Can you work these out from the model? Positions are in its coordinate system, mm. A direction names the side the tool comes from. Coordinates: 2 decimals unless noted, no trailing zeros. Use one line per item in the form item = value.
```python
from build123d import *

# Parameters (mm, degrees)
F0_R     = 1.6
F0_R_2   = 1.25
F0_R_3   = 2
F0_R_4   = 3
F1_DEPTH = 3.175


# Not quite as in the source:
# - a feature names something its author has since deleted; it is built from what else it names


with BuildPart() as f1:
    # F0 (on Top) → F1 (new body)
    with BuildSketch(Plane.XY):
        with BuildLine():
            Line((-49.8799999985, 8.89), (-49.8799999985, -63.5))
            Line((-49.8799999985, -63.5), (49.8799999985, -63.5))
            Line((49.8799999985, -63.5), (49.8799999985, 8.89))
            Line((49.8799999985, 8.89), (57.4999999985, 8.89))
            add(Edge.make_bspline(
                [(15.7093216459, 79.3836478465), (17.5511050126, 65.7915878149), (21.2374579051, 38.4486252292), (53.8863670451, 16.0459412112), (57.4999999985, 8.89)],
                knots=[0, 0, 0, 0, 0.4099092451, 0.8244764195, 0.8244764195, 0.8244764195, 0.8244764195], degree=3))
            ThreePointArc((15.7093216459, 79.3836478465), (0, 91.6600956823), (-15.7093216459, 79.3836478465))
            add(Edge.make_bspline(
                [(-15.7093216459, 79.3836478465), (-15.8351413169, 78.4551192516), (-15.960918893, 77.5265804672), (-16.0889396188, 76.5984215036)],
                knots=[0, 0, 0, 0, 0.0280025584, 0.0280025584, 0.0280025584, 0.0280025584], degree=3))
            add(Edge.make_bspline(
                [(-16.0889396188, 76.5984215036), (-17.8349219122, 63.9399312026), (-22.3463470917, 37.6877393462), (-53.8863670451, 16.0459412112), (-57.4999999985, 8.89)],
                knots=[0.0280025584, 0.0280025584, 0.0280025584, 0.0280025584, 0.4099092451, 0.8244764195, 0.8244764195, 0.8244764195, 0.8244764195], degree=3))
            Line((-57.4999999985, 8.89), (-49.8799999985, 8.89))
        make_face()
        with Locations((-40.5299999985, -54.15)):
            Circle(F0_R, mode=Mode.SUBTRACT)
        with Locations((-40.5299999985, -3.635)):
            Circle(F0_R, mode=Mode.SUBTRACT)
        with Locations((-8, -12)):
            Circle(F0_R_2, mode=Mode.SUBTRACT)
        with Locations((40.5299999985, -54.15)):
            Circle(F0_R, mode=Mode.SUBTRACT)
        with Locations((0, -20)):
            Circle(F0_R_2, mode=Mode.SUBTRACT)
        with Locations((0, -12)):
            Circle(F0_R_3, mode=Mode.SUBTRACT)
        with Locations((8, -12)):
            Circle(F0_R_2, mode=Mode.SUBTRACT)
        with Locations((0, -4)):
            Circle(F0_R_2, mode=Mode.SUBTRACT)
        with Locations((40.5299999985, -3.635)):
            Circle(F0_R, mode=Mode.SUBTRACT)
        with BuildLine():
            Line((-21.7048343448, 33.51030308), (-4.9567933963, 18.14211905))
            Line((-4.9567933963, 18.14211905), (-17.3775311559, -3.8353991695))
            Line((-17.3775311559, -3.8353991695), (-43.0274941027, 6.520065479))
            ThreePointArc((-43.0274941027, 6.520065479), (-32.1093228463, 19.8122760508), (-21.7048343448, 33.51030308))
        make_face(mode=Mode.SUBTRACT)
        with BuildLine():
            ThreePointArc((-10.4206144746, 63.5413418448), (-7.8378238948, 61.7519957694), (-4.9567933963, 60.4981098798))
            Line((-4.9567933963, 60.4981098798), (-4.9567933963, 29.0021225758))
            Line((-4.9567933963, 29.0021225758), (-17.2076895833, 40.2436777949))
            ThreePointArc((-17.2076895833, 40.2436777949), (-13.397490451, 51.7711279758), (-10.4206144746, 63.5413418448))
        make_face(mode=Mode.SUBTRACT)
        with Locations((-0.0292583045, 76.2)):
            Circle(F0_R_4, mode=Mode.SUBTRACT)
        with BuildLine():
            Line((17.3775311559, -3.8353991695), (4.9567933963, 18.14211905))
            Line((4.9567933963, 18.14211905), (21.7048343448, 33.51030308))
            ThreePointArc((21.7048343448, 33.51030308), (32.1093228463, 19.8122760508), (43.0274941027, 6.520065479))
            Line((43.0274941027, 6.520065479), (17.3775311559, -3.8353991695))
        make_face(mode=Mode.SUBTRACT)
        with BuildLine():
            Line((17.2076895833, 40.2436777949), (4.9567933963, 29.0021225758))
            Line((4.9567933963, 29.0021225758), (4.9567933963, 60.4981098798))
            ThreePointArc((4.9567933963, 60.4981098798), (7.8378238948, 61.7519957694), (10.4206144746, 63.5413418448))
            ThreePointArc((10.4206144746, 63.5413418448), (13.397490451, 51.7711279758), (17.2076895833, 40.2436777949))
        make_face(mode=Mode.SUBTRACT)
    extrude(amount=F1_DEPTH)


solid = f1.part
```
Q1. Thinking about a two-plate mould opening in Y: for faces 4 (the flat face through (49.88, -28, 2)), 5 (the flat face through (-1, -63.5, 2)), 6 (the cylindrical face through (-7.876, 61.773, 1.565)), which applies, released by +Y, released by -Y, zero draft, split by the parting line, or undercut?
Return value:
face_4 = zero draft
face_5 = released by -Y
face_6 = undercut
Q2. Will these pins go through, and if not, where does the flat tip stop? pin 1 (1.6 mm diameter, centred on y = 42, z = 1.5, fed in from -X); pin 2 (2.5 mm diameter, centred on x = 0, y = -12, fed in from +Z).
Return value:
pin_1 = -27.41
pin_2 = through
Q3. Suppose I cut it at A-A (y = 12.5). Give the number of separate pieces and of enclosed holes in the cut face, then the cut area to 3 significant figures.
Return value:
separate_pieces = 3
enclosed_holes = 0
area = 159 mm2
Q4. For faces 1 (the flat face through (30.382, 1.415, 1.565)), 2 (the flat face through (-54, 8.89, 2)), 3 (the flat face through (-1, -2, 3.175)), which set-ups out of +Z, -Z, +X, -X, +Y, -Y let a thin tool reach every point of the face, with its end or its side?
Return value:
face_1 = +Z, -Z
face_2 = +Z, -Z, -X, -Y
face_3 = +Z, +X, -X, +Y, -Y
Q5. If I drill on line 1 (Y direction, x = 0, z = 1.8); line 2 (X direction, y = -54, z = 2.3); line 3 (X direction, y = -3.5, z = 0.25), over which ranges is the centre line in solid material (lowest first)? Write a range as from..to.
Return value:
line_1 = -63.5..-21.25, -18.75..-14, -10..-5.25, -2.75..73.2, 79.2..91.66
line_2 = -49.88..-42.12, -38.94..38.94, 42.12..49.88
line_3 = -49.88..-42.12, -38.94..-18.21, -17.19..-1.15, 1.15..17.19, 18.21..38.94, 42.12..49.88
